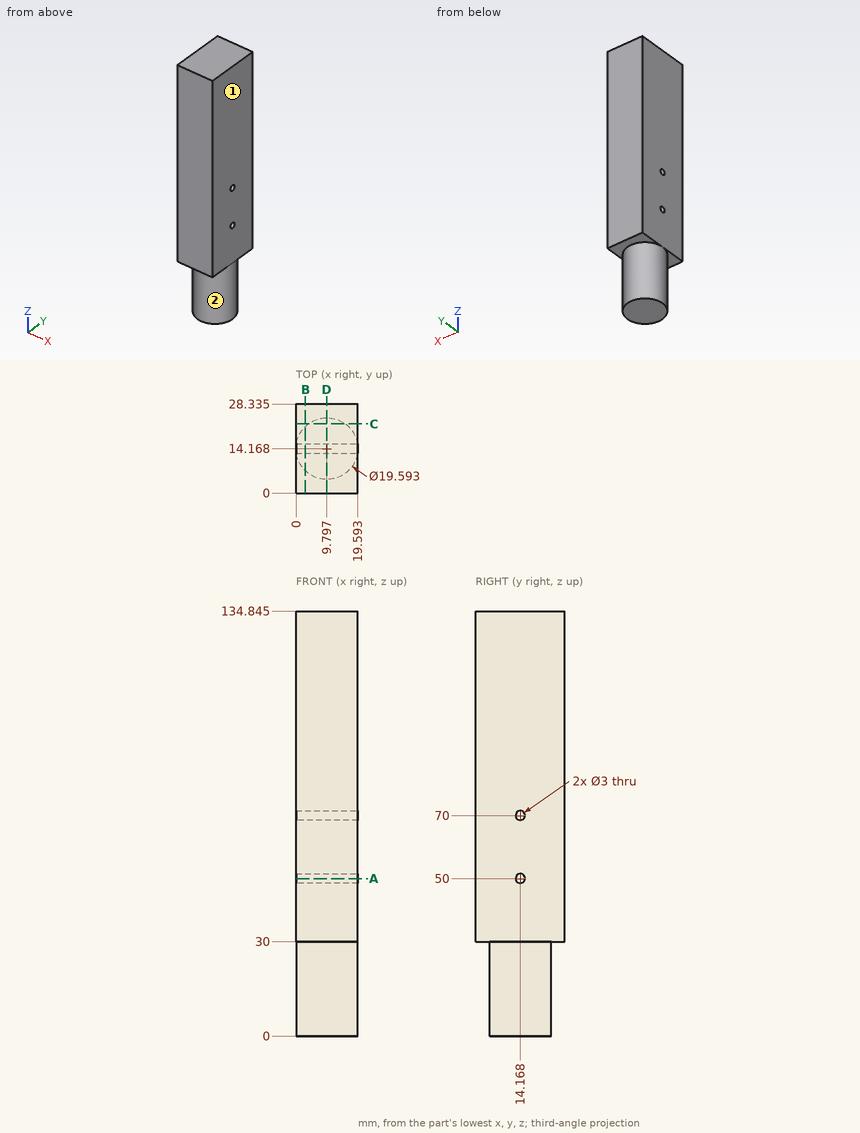
Answer from the drawing. Dimensions are ordinates in mm from the lowest x, y and z of the part. A direction names the side the tool comes from. Coordinates: 2 decimals unless noted, no trailing zeros. Write each loop counter-clockwise with the first axis right and the second up, starting at its lowest first coordinate (ties: lowest second). Pieces come first, ordered by that corner, then holes. Notation, with made-up numbers: (72.25, 9) - (117.25, 9) arc R31 cw to (117.25, 42) - close; hole circle Ø10 at (-28.5, 46). An arc over 180 degrees is marked (long way). Return JSON: item names as keys, results as strings.
1. Consider line 1 along Y through (x, z) = (8.5, 70) (1 decimal); line 2 along Z through (x, y) = (9, 15) (1 decimal); line 3 along Z through (x, y) = (1.25, 13.75) (1 decimal). Determine where each line is inside the solid, lowest interval first.
Final values:
{"line 1": "0 to 12.7, 15.7 to 28.3", "line 2": "0 to 48.8, 51.2 to 68.8, 71.2 to 134.8", "line 3": "0 to 48.6, 51.4 to 68.6, 71.4 to 134.8"}
2. The part is cut by section D-D on x = 9.75. Determine the outline of the cut face in (y, z) (1 decimal), then the cut area to 3 significant figures.
Final values:
{"outline": "(0, 30) - (4.4, 30) - (4.4, 0) - (24, 0) - (24, 30) - (28.3, 30) - (28.3, 134.8) - (0, 134.8) - close; hole circle Ø3 at (14.2, 50); hole circle Ø3 at (14.2, 70)", "area": "3,540 mm^2"}
3. The part is cut by section A-A on z = 50. Determine the outline of the cut face in (x, y) (1 decimal).
Final values:
{"outline": "(0, 0) - (19.6, 0) - (19.6, 12.7) - (0, 12.7) - close; (0, 15.7) - (19.6, 15.7) - (19.6, 28.3) - (0, 28.3) - close"}
4. Which of the six approach directions +Z, -Z, +X, -X, +Y, -Y give full straight-line access (tool end or side, diameter ignored) to the marked faces 1 and 2?
Final values:
{"face 1": "+Z, -Z, +X, +Y, -Y", "face 2": "-Z"}
5. The part is cut by section C-C on y = 22. Determine the outline of the cut face in (x, z) (1 decimal), then the cut area to 3 significant figures.
Final values:
{"outline": "(0, 30) - (3.9, 30) - (3.9, 0) - (15.7, 0) - (15.7, 30) - (19.6, 30) - (19.6, 134.8) - (0, 134.8) - close", "area": "2,410 mm^2"}
6. Each of these flat-tipped pins is pushed along its axis until it touches: pin 1 Ø8 at (x, z) = (9.5, 20) entering from -Y; pin 2 Ø10 at (x, z) = (11, 13.5) entering from +Y. Where does it stop, or does it pass through?
Final values:
{"pin 1": "y = 4.37", "pin 2": "y = 23.96"}
7. The part is cut by section B-B on x = 3. Determine the outline of the cut face in (y, z) (1 decimal).
Final values:
{"outline": "(0, 30) - (7.1, 30) - (7.1, 0) - (21.2, 0) - (21.2, 30) - (28.3, 30) - (28.3, 134.8) - (0, 134.8) - close; hole circle Ø3 at (14.2, 50); hole circle Ø3 at (14.2, 70)"}
